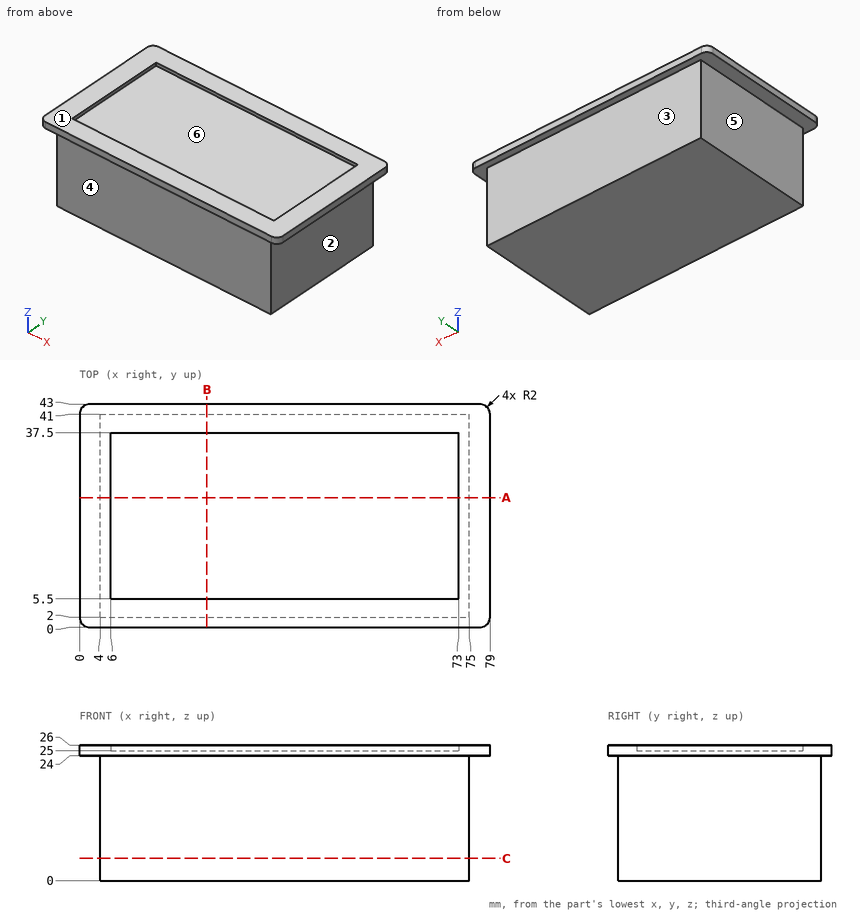
Geometry check sheet. Reference: drawing and pictorial views, mm from the part's lowest x, y, z. A direction names the side the tool comes from. Give positions to 0.01 mm unless a question says otherwise; leave off trailing zeros. Order: outer loops, then holes, each group sorted by start corner. A loop starts at its lowest first (then second) coordinate and runs counter-clockwise, first axis right, second up. Notation, with made-up numbers: M 54.25,59.5 L 83.25,59.5 A22 ccw 83.25,69.5 Z; hole C 57.25,66.25 d9. An arc over 180 degrees is marked long. Return JSON: item names as keys, results as strings. Group by question number.
1) Section check B-B on x = 24.5. Record the cut outline in (y, z).
2) Access from +Z, -Z, +X, -X, +Y, -Y to the whole of each face (thin tool, end or side, straight path). Record for the marked faces 1, 2 and 3.
3) Go/stop test with flat-tipped pins: pin 1 Ø4 at (y, z) = (24, 3) entering from +X; pin 2 Ø12 at (x, y) = (57, 25.5) entering from +Z; pin 3 Ø8 at (x, z) = (70.5, 5) entering from +Y. Record where each tip stops, or that it passes through.
4) Section check C-C on z = 4.25. Record the cut outline in (x, y).
5) Scan lines: line 1 (Y direction, x = 7, z = 4); line 2 (Z direction, x = 50, y = 34); line 3 (X direction, y = 18.5, z = 16.75). Record each from-to range of solid material in increasing order.
6) Section check A-A on y = 25. Record the cut outline in (x, z), and give its area (4 significant figures).
7) Mould release check, pull along X, two halves, no side actions. Record for the marked faces 4, 5 and 6: pulls with the +X half, pulls with the -X half, needs draft (parallel to the pull), parting line crosses it, or undercut.
Answer block:
{
 "1": {"outline": "M 0,24 L 2,24 L 2,0 L 41,0 L 41,24 L 43,24 L 43,26 L 37.5,26 L 37.5,25 L 5.5,25 L 5.5,26 L 0,26 Z"},
 "2": {"face 1": "+Z, +X, -X, +Y, -Y", "face 2": "-Z, +X, +Y, -Y", "face 3": "-Z, +X, -X, +Y"},
 "3": {"pin 1": "stops at x = 75", "pin 2": "stops at z = 25", "pin 3": "stops at y = 41"},
 "4": {"outline": "M 4,2 L 75,2 L 75,41 L 4,41 Z"},
 "5": {"line 1": "y = 2 to 41", "line 2": "z = 0 to 25", "line 3": "x = 4 to 75"},
 "6": {"outline": "M 0,24 L 4,24 L 4,0 L 75,0 L 75,24 L 79,24 L 79,26 L 73,26 L 73,25 L 6,25 L 6,26 L 0,26 Z", "area": "1,795 mm^2"},
 "7": {"face 4": "needs draft", "face 5": "pulls with the -X half", "face 6": "undercut"}
}
